```python
from build123d import *

# Parameters (mm, degrees)
SKETCH1_R                                  = 3.175
BOSS_EXTRUDE1_DEPTH                        = 3.175
SKETCH3_W                                  = 1.27
SKETCH3_H                                  = 6.721052908
CUT_EXTRUDE1_DEPTH                         = 3.175
SKETCH4_R                                  = 0.79375
CUT_EXTRUDE2_DEPTH                         = 9.89
SKETCH5_R                                  = 0.762
BOSS_EXTRUDE2_DEPTH                        = 3.175
MIRROR1_AT_THE_SECOND_PLANE_COPY_1_SKETC_R = 0.762
MIRROR1_AT_THE_SECOND_PLANE_COPY_1_DEPTH   = 3.175


with BuildPart() as part:
    # Sketch1 → Boss-Extrude1 (new body)
    with BuildSketch(Plane(origin=(0, 0, 0), x_dir=(1, 0, 0), z_dir=(0, 1, 0))):
        with BuildLine():
            Line((3.175, 4.751904881), (3.175, 9.831904881))
            Line((3.175, 9.831904881), (-3.175, 9.831904881))
            Line((-3.175, 9.831904881), (-3.175, 4.751904881))
            ThreePointArc((-3.175, 4.751904881), (0, -5.715), (3.175, 4.751904881))
        make_face()
        Circle(SKETCH1_R, mode=Mode.SUBTRACT)
    extrude(amount=BOSS_EXTRUDE1_DEPTH)

    # Sketch3 → Cut-Extrude1 (cut)
    with BuildSketch(Plane(origin=(0, 3.175, 0), x_dir=(1, 0, 0), z_dir=(0, 1, 0))):
        with Locations((0, 6.471378427)):
            Rectangle(SKETCH3_W, SKETCH3_H)
    extrude(amount=-CUT_EXTRUDE1_DEPTH, mode=Mode.SUBTRACT)

    # Sketch4 → Cut-Extrude2 (cut, through all)
    with BuildSketch(Plane(origin=(3.175, 0, 0), x_dir=(0, 0, -1), z_dir=(1, 0, 0))):
        with Locations((7.926904881, 1.5875)):
            Circle(SKETCH4_R)
    extrude(amount=-CUT_EXTRUDE2_DEPTH, mode=Mode.SUBTRACT)

    # Sketch5 → Boss-Extrude2 (add)
    with BuildSketch(Plane.XZ):
        with BuildLine():
            Line((-4.176191145, -5.579356164), (-3.278165533, -4.681330552))
            ThreePointArc((-3.278165533, -4.681330552), (-4.041115254, -4.041115254), (-4.681330552, -3.278165533))
            Line((-4.681330552, -3.278165533), (-5.579356164, -4.176191145))
            ThreePointArc((-5.579356164, -4.176191145), (-5.579356164, -5.579356164), (-4.176191145, -5.579356164))
        make_face()
        with Locations((-4.877773655, -4.877773655)):
            Circle(SKETCH5_R, mode=Mode.SUBTRACT)
    boss_extrude2 = extrude(amount=-BOSS_EXTRUDE2_DEPTH)

    # Mirror1: Boss-Extrude2 across plane
    add(boss_extrude2.mirror(Plane(origin=(0, 0, 0), x_dir=(0, 0, 1), z_dir=(1, 0, 0))))

    # Mirror1 at the second plane: Boss-Extrude2 across plane
    add(boss_extrude2.mirror(Plane.XY))

    # Mirror1 at the second plane copy 1 sketc → Mirror1 at the second plane copy 1 (add)
    with BuildSketch(Plane(origin=(0, 0, 0), x_dir=(-1, 0, 0), z_dir=(0, -1, 0))):
        with BuildLine():
            Line((-4.176191145, -5.579356164), (-3.278165533, -4.681330552))
            ThreePointArc((-3.278165533, -4.681330552), (-4.041115254, -4.041115254), (-4.681330552, -3.278165533))
            Line((-4.681330552, -3.278165533), (-5.579356164, -4.176191145))
            ThreePointArc((-5.579356164, -4.176191145), (-5.579356164, -5.579356164), (-4.176191145, -5.579356164))
        make_face()
        with Locations((-4.877773655, -4.877773655)):
            Circle(MIRROR1_AT_THE_SECOND_PLANE_COPY_1_SKETC_R, mode=Mode.SUBTRACT)
    extrude(amount=-MIRROR1_AT_THE_SECOND_PLANE_COPY_1_DEPTH)


solid = part.part
```
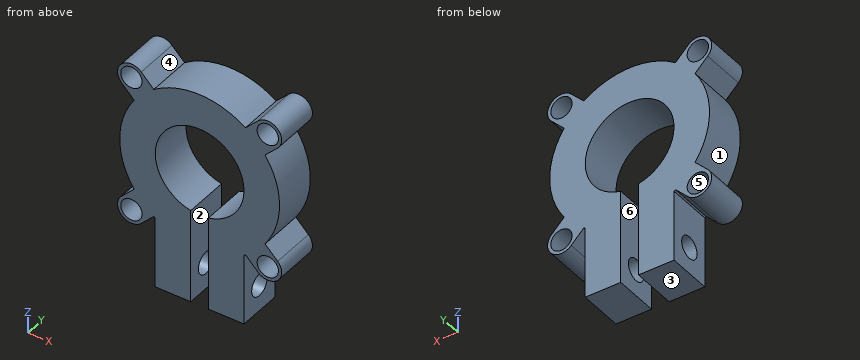
Model file for the job. Use its own axes, mm. Face numbers are marked on the shaded views. A direction names the side the tool comes from. Coordinates: 2 decimals unless noted, no trailing zeros. Order: outer loops, then holes, each group sorted by start corner. A loop starts at its lowest first (then second) coordinate and runs counter-clockwise, first axis right, second up. Notation, with made-up numbers: (59, 38) -> (71, 38) arc R34 cw to (71, 71) -> close; hole circle Ø10 at (79.5, 65.5). An arc over 180 degrees is marked (long way). Answer as a JSON object with one key per item and string values. Group by question number.
1) Cut at B-B, the plane z = 0. Write the cut outline in (x, y) (3 decimals), then the cut area to 3 significant figures.
2) Cut at C-C, the plane z = -4.5. Write the cut outline in (x, y) (3 decimals).
3) Which spindle directions (+Z, -Z, +X, -X, +Y, -Y) get a long thin tool onto all of the face, cutting with end or side? Do the marked faces 4, 5 and 6. Say none if no direction does.
4) Drill centre lines: L1, parallel to X at y = 1.1, z = -5 (3 decimals); L2, parallel to X at y = 1.05, z = -6.75 (3 decimals); L3, parallel to Z at x = -2.5, y = 1.7. Where is each one in solid material? Low to high.
5) Cut at D-D, the plane x = 3. Write the cut outline in (y, z) (1 decimal).
6) Flat gauge pins, fed straight in: pin 1 (1 mm diameter, centred on y = 2, z = 4, fed in from -X); pin 2 (2 mm diameter, centred on x = -4.88, z = -4.88, fed in from +Y) (3 decimals); pin 3 (1.6 mm diameter, centred on y = 2, z = -7, fed in from +X) (3 decimals); pin 4 (1.6 mm diameter, centred on y = 1, z = -8.5, fed in from -X) (3 decimals). Where does each tip first touch, or does it go through?
7) Cut at A-A, the plane x = -2.5. Write the cut outline in (y, z) (1 decimal), then the cut area to 3 significant figures.
8) Pull direction X, two halves, no side cores. Call the marked faces 1, 2 and 3: +X half, -X half, draft (parallel to the pull), parting line (faces both ways), or undercut.
Check values:
{
 "1": {"outline": "(-5.715, 0) -> (-3.175, 0) -> (-3.175, 3.175) -> (-5.715, 3.175) -> close; (3.175, 0) -> (5.715, 0) -> (5.715, 3.175) -> (3.175, 3.175) -> close", "area": "16.1 mm²"},
 "2": {"outline": "(-5.795, 0) -> (-5.54, 0) -> (-5.54, 3.175) -> (-5.795, 3.175) -> close; (-4.216, 0) -> (-0.635, 0) -> (-0.635, 3.175) -> (-4.216, 3.175) -> close; (0.635, 0) -> (4.216, 0) -> (4.216, 3.175) -> (0.635, 3.175) -> close; (5.54, 0) -> (5.795, 0) -> (5.795, 3.175) -> (5.54, 3.175) -> close"},
 "3": {"face 4": "+Z, +Y, -Y", "face 5": "+Y, -Y", "face 6": "-Z, +Y, -Y"},
 "4": {"L1": "x = -5.862 to -5.63, -4.126 to -3.597, -3.175 to -0.635, 0.635 to 3.175, 3.597 to 4.126, 5.63 to 5.862", "L2": "x = -3.175 to -0.635, 0.635 to 3.175", "L3": "z = -9.83 to -8.71, -7.14 to -1.96, 1.96 to 5.14"},
 "5": {"outline": "(0, -9.8) -> (3.2, -9.8) -> (3.2, -1) -> (0, -1) -> close; (0, 1) -> (3.2, 1) -> (3.2, 4.9) -> (0, 4.9) -> close; hole circle Ø1.6 at (1.6, -7.9)"},
 "6": {"pin 1": "stops at x = -5.8", "pin 2": "stops at y = 3.175", "pin 3": "stops at x = 3.175", "pin 4": "stops at x = -3.175"},
 "7": {"outline": "(0, -9.8) -> (3.2, -9.8) -> (3.2, -2) -> (0, -2) -> close; (0, 2) -> (3.2, 2) -> (3.2, 5.1) -> (0, 5.1) -> close; hole circle Ø1.6 at (1.6, -7.9)", "area": "33.1 mm²"},
 "8": {"face 1": "-X half", "face 2": "undercut", "face 3": "draft"}
}
